from build123d import *

# Parameters (mm, degrees)
SKETCH1_R          = 2
BASE_DEPTH         = 7
WALLS_START        = 7
SKETCH1_3_R        = 1.6
WALLS_DEPTH        = 23
STANDOFFS_START    = 7
SKETCH1_4_R        = 3.6
SKETCH1_4_R_2      = 1.6
STANDOFFS_DEPTH    = 3
INTERNAL_FILLET_R  = 3
EXTERNAL_FILLET_R  = 3
SKETCH2_R          = 8
CUT_EXTRUDE1_DEPTH = 2


with BuildPart() as part:
    # Sketch1 → BASE (new body)
    with BuildSketch(Plane(origin=(0, 0, 0), x_dir=(1, 0, 0), z_dir=(0, 1, 0))):
        Polygon((-31.75, -38.07), (-37.75, -38.07), (-37.75, -44.07), (-31.75, -44.07), (-31.75, -54.07), (31.75, -54.07), (31.75, -44.07), (37.75, -44.07), (37.75, -38.07), (31.75, -38.07), (31.75, 38.07), (37.75, 38.07), (37.75, 44.07), (31.75, 44.07), (31.75, 54.07), (-31.75, 54.07), (-31.75, 44.07), (-37.75, 44.07), (-37.75, 38.07), (-31.75, 38.07), align=None)
        with Locations(Location((-34.75, -41.07, 0), (0, 0, 270))):
            Circle(SKETCH1_R, mode=Mode.SUBTRACT)
        with Locations(Location((-34.75, 41.07, 0), (0, 0, 270))):
            Circle(SKETCH1_R, mode=Mode.SUBTRACT)
        with Locations(Location((34.75, -41.07, 0), (0, 0, 270))):
            Circle(SKETCH1_R, mode=Mode.SUBTRACT)
        with Locations(Location((34.75, 41.07, 0), (0, 0, 270))):
            Circle(SKETCH1_R, mode=Mode.SUBTRACT)
    extrude(amount=BASE_DEPTH)

    # Sketch1<3> → Walls (add)
    with BuildSketch(Plane(origin=(0, 0, 0), x_dir=(1, 0, 0), z_dir=(0, 1, 0)).offset(WALLS_START)):
        Polygon((-31.75, 38.07), (-31.75, -38.07), (-31.75, -44.07), (-31.75, -54.07), (31.75, -54.07), (31.75, -44.07), (31.75, -38.07), (31.75, 38.07), (31.75, 44.07), (31.75, 54.07), (-31.75, 54.07), (-31.75, 44.07), align=None)
        with Locations(Location((-28.15, -50.47, 0), (0, 0, 270))):
            Circle(SKETCH1_3_R, mode=Mode.SUBTRACT)
        with BuildLine():
            Line((24.925096901, -52.07), (-24.925096901, -52.07))
            ThreePointArc((-24.925096901, -52.07), (-25.604415588, -47.924415588), (-29.75, -47.245096901))
            Line((-29.75, -47.245096901), (-29.75, 47.245096901))
            ThreePointArc((-29.75, 47.245096901), (-25.604415588, 47.924415588), (-24.925096901, 52.07))
            Line((-24.925096901, 52.07), (24.925096901, 52.07))
            ThreePointArc((24.925096901, 52.07), (25.604415588, 47.924415588), (29.75, 47.245096901))
            Line((29.75, 47.245096901), (29.75, -47.245096901))
            ThreePointArc((29.75, -47.245096901), (25.604415588, -47.924415588), (24.925096901, -52.07))
        make_face(mode=Mode.SUBTRACT)
        with Locations(Location((28.15, -50.47, 0), (0, 0, 270))):
            Circle(SKETCH1_3_R, mode=Mode.SUBTRACT)
        with Locations(Location((-28.15, 50.47, 0), (0, 0, 270))):
            Circle(SKETCH1_3_R, mode=Mode.SUBTRACT)
        with Locations(Location((28.15, 50.47, 0), (0, 0, 270))):
            Circle(SKETCH1_3_R, mode=Mode.SUBTRACT)
    extrude(amount=WALLS_DEPTH)

    # Sketch1<4> → Standoffs (add)
    # profile 1 of 2: a face of its own
    with BuildSketch(Plane(origin=(0, 0, 0), x_dir=(1, 0, 0), z_dir=(0, 1, 0)).offset(STANDOFFS_START)):
        with Locations(Location((0, 42.07, 0), (0, 0, 270))):
            Circle(SKETCH1_4_R)
        with Locations(Location((0, 42.07, 0), (0, 0, 270))):
            Circle(SKETCH1_4_R_2, mode=Mode.SUBTRACT)
    # profile 2 of 2: a face of its own
    with BuildSketch(Plane(origin=(0, 0, 0), x_dir=(1, 0, 0), z_dir=(0, 1, 0)).offset(STANDOFFS_START)):
        with Locations(Location((0, -31.63, 0), (0, 0, 270))):
            Circle(SKETCH1_4_R)
        with Locations(Location((0, -31.63, 0), (0, 0, 270))):
            Circle(SKETCH1_4_R_2, mode=Mode.SUBTRACT)
    extrude(amount=STANDOFFS_DEPTH)

    # Internal Fillet
    internal_fillet_edges = [part.edges().sort_by_distance(p)[0] for p in [
        (-29.75, 18.5, 47.245096901),
        (-25.604415588, 7, 47.924415588),
        (-24.925096901, 18.5, 52.07),
        (0, 7, 52.07),
        (24.925096901, 18.5, 52.07),
        (25.604415588, 7, 47.924415588),
        (29.75, 18.5, 47.245096901),
        (29.75, 7, 0),
        (29.75, 18.5, -47.245096901),
        (25.604415588, 7, -47.924415588),
        (24.925096901, 18.5, -52.07),
        (-24.925096901, 18.5, -52.07),
        (-25.604415588, 7, -47.924415588),
        (-29.75, 18.5, -47.245096901),
        (0, 7, -45.67),
        (0, 7, 28.03),
        (-29.75, 7, 0),
        (0, 7, -52.07),
    ]]
    fillet(internal_fillet_edges, radius=INTERNAL_FILLET_R - 0.0001)  # a hair under: the kernel refuses the full size

    # External Fillet
    external_fillet_edges = [part.edges().sort_by_distance(p)[0] for p in [
        (-31.75, 15, 54.07),
        (-31.75, 15, -54.07),
        (31.75, 15, -54.07),
        (31.75, 15, 54.07),
        (31.75, 3.5, 38.07),
        (37.75, 3.5, 38.07),
        (37.75, 3.5, 44.07),
        (31.75, 3.5, 44.07),
        (31.75, 3.5, -38.07),
        (31.75, 3.5, -44.07),
        (37.75, 3.5, -38.07),
        (37.75, 3.5, -44.07),
        (-31.75, 3.5, -38.07),
        (-37.75, 3.5, -38.07),
        (-37.75, 3.5, -44.07),
        (-31.75, 3.5, -44.07),
        (-31.75, 3.5, 38.07),
        (-37.75, 3.5, 38.07),
        (-37.75, 3.5, 44.07),
        (-31.75, 3.5, 44.07),
    ]]
    fillet(external_fillet_edges, radius=EXTERNAL_FILLET_R - 0.0001)  # a hair under: the kernel refuses the full size

    # Sketch2 → Cut-Extrude1 (cut)
    with BuildSketch(Plane(origin=(27.4, 0, 54.07), x_dir=(-1, 0, 0), z_dir=(0, 0, -1))):
        with Locations(Location((27.4, 19.200000012, 0), (0, 0, 180))):
            Circle(SKETCH2_R)
    extrude(amount=CUT_EXTRUDE1_DEPTH, mode=Mode.SUBTRACT)


solid = part.part
Source: CAD feature listing. Evaluate the final solid. Frame: model axes, mm. A direction names the side the tool comes from. Coordinates: 2 decimals unless noted, no trailing zeros. Order: outer loops, then holes, each group sorted by start corner. A loop starts at its lowest first (then second) coordinate and runs counter-clockwise, first axis right, second up. Notation, with made-up numbers: M -27.75,-15.75 L 30.25,-15.75 A13 cw 30.25,-3.75 Z; hole C 33,24 d2. An arc over 180 degrees is marked long. Write each question's results on one line, items separated by ' | '. Start each with the question number.
1. Draft query along Z for faces 1 (the face through (32.61, 3.55, 44.97)), 2 (the face through (-1, 0, -1)), 3 (the face through (-29.068, 20.14, 45.925)). Return one class per face: +Z half, -Z half, draft (parallel to the pull), parting line (faces both ways), or undercut.
2. Pin query (flat end, axial travel): pin 1 (6 mm diameter, centred on y = 12, z = 3, fed in from -X); pin 2 (3.5 mm diameter, centred on x = 0, z = -42.07, fed in from +Y); pin 3 (1.6 mm diameter, centred on x = 28, z = -50, fed in from +Y). Return the tip coordinate at first contact, or that it passes through.
3. Section D-D, the plane x = -20. Return the cut outline in (y, z), then the cut area to 3 significant figures.
4. Section C-C, the plane y = 15. State how many separate pieces and enclosed holes the cut face has, then the cut area to 3 significant figures.
5. Reachability of faces 4 (the face through (32.61, 3.55, -37.17)), 5 (the face through (-36.85, 3.55, 38.93)), 6 (the face through (32.5, 7, -40.7)), 7 (the face through (-31, 30, -12)), 8 (the face through (-25.625, 19.86, -47.904)) from +Z, -Z, +X, -X, +Y, -Y: full face, straight path, thin tool, end or side. Return the list, or none.
6. Section B-B, the plane z = 15. Return the cut outline in (x, y).
7. Material intervals for L1, parallel to X at y = 5.25, z = 41.07; L2, parallel to Z at x = -20, y = 24; L3, parallel to X at y = 15.5, z = 20, sorted ascending.
Solution:
1) face 1: +Z half | face 2: draft | face 3: undercut
2) pin 1: x = -31.75 | pin 2: y = 10 | pin 3: y = 7
3) outline: M 0,-54.07 L 30,-54.07 L 30,-52.07 L 10,-52.07 A3 cw 7,-49.07 L 7,49.07 A3 cw 10,52.07 L 30,52.07 L 30,54.07 L 0,54.07 Z | area: 853 mm²
4) separate pieces: 1 | enclosed holes: 4 | area: 713 mm²
5) face 4: +X, +Y, -Y | face 5: -X, +Y, -Y | face 6: +Z, -Z, +X, +Y | face 7: +Z, -Z, +X, -X, +Y | face 8: +Y
6) outline: M -31.75,0 L 31.75,0 L 31.75,30 L 29.75,30 L 29.75,10 A3 cw 26.75,7 L -26.75,7 A3 cw -29.75,10 L -29.75,30 L -31.75,30 Z
7) L1: -37.75 to -36.75, -32.75 to 32.75, 36.75 to 37.75 | L2: -54.07 to -52.07, 52.07 to 54.07 | L3: -31.75 to -29.75, 29.75 to 31.75
